Part model, mm, in its own coordinate system. A direction names the side the tool comes from. Round coordinates to 2 decimals unless told otherwise and drop trailing zeros. Write each loop counter-clockwise with the first axis right and the second up, starting at its lowest first coordinate (ties: lowest second). Pieces come first, ordered by that corner, then holes.
1) Saw through at C-C on y = -1.5. Write the cut outline in (x, z).
2) Drill centre lines: L1, parallel to Z at x = 5.75, y = -2.5; L2, parallel to X at y = -0.25, z = -2; L3, parallel to Y at x = -6.5, z = 7.5. Where is each one in solid material? Low to high.
3) Saw through at D-D on z = -1.5. Write the cut outline in (x, y).
4) Flat gauge pins, fed straight in: pin 1 (4 mm diameter, centred on x = -0.5, z = -13, fed in from -Y); pin 2 (1.5 mm diameter, centred on y = 0, z = -11, fed in from +X); pin 3 (1 mm diameter, centred on y = -5, z = -5, fed in from -X). Where does each tip first touch, or does it go through?
5) Which spindle directions (+Z, -Z, +X, -X, +Y, -Y) get a long thin tool onto all of the face, cutting with end or side? Do faces 1 (the flat face through (0, 0, 10)), 2 (the cylindrical face through (-5, 0, -4)). Say none if no direction does.
6) Saw through at A-A on z = 4. Write the cut outline in (x, y).
7) Saw through at B-B on x = 0. Write the cut outline in (y, z), and give its area (3 significant figures).
```python
from build123d import *

# Parameters (mm, degrees)
EXTRUDE_1_DEPTH     = 10
SKETCH_3_R          = 4.5
SKETCH_3_R_2        = 2.5
EXTRUDE_2_DEPTH     = 120
SKETCH_5_R          = 5
SKETCH_5_R_2        = 4.5
EXTRUDE_3_DEPTH     = 45
SKETCH_6_R          = 4.5
SKETCH_6_R_2        = 2.5
EXTRUDE_5_DEPTH     = 25
CUT_EXTRUDE_START   = -100
SKETCH_7_R          = 4.5
CUT_EXTRUDE_1_DEPTH = 100
CUT_EXTRUDE_START_2 = -33
SKETCH_9_R          = 5
CUT_EXTRUDE_2_DEPTH = 33
SKETCH_8_R          = 4.5
EXTRUDE_6_DEPTH     = 29
CUT_EXTRUDE_START_3 = -4
SKETCH_10_R         = 5
SKETCH_10_R_2       = 4.5
CUT_EXTRUDE_3_DEPTH = 4


with BuildPart() as part:
    # 草图1 → 凸台-拉伸1 (new body)
    with BuildSketch(Plane.XY):
        Polygon((8, 0), (4, 6.92820323), (-4, 6.92820323), (-8, 0), (-4, -6.92820323), (4, -6.92820323), align=None)
    extrude(amount=EXTRUDE_1_DEPTH)

    # 草图3 → 凸台-拉伸2 (add)
    with BuildSketch(Plane(origin=(0, 0, 0), x_dir=(-1, 0, 0), z_dir=(0, 0, -1))):
        with Locations(Location((0, 0, 0), (0, 0, 180))):
            Circle(SKETCH_3_R)
        Circle(SKETCH_3_R_2, mode=Mode.SUBTRACT)
    extrude(amount=EXTRUDE_2_DEPTH)

    # 草图5 → 凸台-拉伸3 (add)
    with BuildSketch(Plane(origin=(0, 0, 0), x_dir=(-1, 0, 0), z_dir=(0, 0, -1))):
        with Locations(Location((0, 0, 0), (0, 0, 180))):
            Circle(SKETCH_5_R)
        Circle(SKETCH_5_R_2, mode=Mode.SUBTRACT)
    extrude(amount=EXTRUDE_3_DEPTH)

    # 草图6 → 凸台-拉伸5 (add)
    with BuildSketch(Plane(origin=(0, 0, -120), x_dir=(-1, 0, 0), z_dir=(0, 0, -1))):
        Circle(SKETCH_6_R)
        Circle(SKETCH_6_R_2, mode=Mode.SUBTRACT)
    extrude(amount=EXTRUDE_5_DEPTH)

    # 草图7 → 切除-拉伸1 (cut)
    with BuildSketch(Plane(origin=(0, 0, -145), x_dir=(-1, 0, 0), z_dir=(0, 0, -1)).offset(CUT_EXTRUDE_START)):
        Circle(SKETCH_7_R)
    extrude(amount=CUT_EXTRUDE_1_DEPTH, mode=Mode.SUBTRACT)

    # 草图9 → 切除-拉伸2 (cut)
    with BuildSketch(Plane(origin=(0, 0, -45), x_dir=(-1, 0, 0), z_dir=(0, 0, -1)).offset(CUT_EXTRUDE_START_2)):
        with Locations(Location((0, 0, 0), (0, 0, 180))):
            Circle(SKETCH_9_R)
    extrude(amount=CUT_EXTRUDE_2_DEPTH, mode=Mode.SUBTRACT)

    # 草图8 → 凸台-拉伸6 (add)
    with BuildSketch(Plane(origin=(0, 0, 0), x_dir=(-1, 0, 0), z_dir=(0, 0, -1))):
        with Locations(Location((0, 0, 0), (0, 0, 180))):
            Circle(SKETCH_8_R)
    extrude(amount=EXTRUDE_6_DEPTH)

    # 草图10 → 切除-拉伸3 (cut)
    with BuildSketch(Plane(origin=(0, 0, -12), x_dir=(-1, 0, 0), z_dir=(0, 0, -1)).offset(CUT_EXTRUDE_START_3)):
        with Locations(Location((0, 0, 0), (0, 0, 180))):
            Circle(SKETCH_10_R)
        with Locations(Location((0, 0, 0), (0, 0, 180))):
            Circle(SKETCH_10_R_2, mode=Mode.SUBTRACT)
    extrude(amount=CUT_EXTRUDE_3_DEPTH, mode=Mode.SUBTRACT)


solid = part.part
```
Completed:
1. outline: (-7.13, 0) - (-4.77, 0) - (-4.77, -8) - (-4.24, -8) - (-4.24, -29) - (4.24, -29) - (4.24, -8) - (4.77, -8) - (4.77, 0) - (7.13, 0) - (7.13, 10) - (-7.13, 10) - close
2. L1: z = 0 to 10
2. L2: x = -4.99 to 4.99
2. L3: y = -2.6 to 2.6
3. outline: circle Ø10 at (0, 0)
4. pin 1: stops at y = -4.5
4. pin 2: stops at x = 4.5
4. pin 3: stops at x = -2.18
5. face 1: +Z, +X, -X, +Y, -Y
5. face 2: -Z
6. outline: (-8, 0) - (-4, -6.93) - (4, -6.93) - (8, 0) - (4, 6.93) - (-4, 6.93) - close
7. outline: (-6.93, 0) - (-5, 0) - (-5, -8) - (-4.5, -8) - (-4.5, -29) - (4.5, -29) - (4.5, -8) - (5, -8) - (5, 0) - (6.93, 0) - (6.93, 10) - (-6.93, 10) - close
7. area: 408 mm2
